```python
from build123d import *

# Parameters (mm, degrees)
SALIENTE_EXTRUIR1_DEPTH = 36.83
CROQUIS2_R              = 1.84
CROQUIS2_W              = 9.91
CROQUIS2_H              = 9.91
CORTAR_EXTRUIR1_DEPTH   = 49.541066699
CROQUIS3_W              = 2.1
CROQUIS3_H              = 17.6
CORTAR_EXTRUIR2_DEPTH   = 50.084125743


with BuildPart() as part:
    # Croquis1 → Saliente-Extruir1 (new body)
    with BuildSketch(Plane(origin=(0, 0, 0), x_dir=(0, 0, -1), z_dir=(1, 0, 0))):
        with BuildLine():
            Line((0, 0), (0, 19))
            ThreePointArc((0, 19), (-0.292893219, 19.707106781), (-1, 20))
            Line((-1, 20), (-5.045, 20))
            ThreePointArc((-5.045, 20), (-5.752106781, 19.707106781), (-6.045, 19))
            Line((-6.045, 19), (-6.045, 2.3725))
            ThreePointArc((-6.045, 2.3725), (-6.337893219, 1.665393219), (-7.045, 1.3725))
            Line((-7.045, 1.3725), (-18.505, 1.3725))
            ThreePointArc((-18.505, 1.3725), (-19.212106781, 1.665393219), (-19.505, 2.3725))
            Line((-19.505, 2.3725), (-19.505, 19))
            ThreePointArc((-19.505, 19), (-19.797893219, 19.707106781), (-20.505, 20))
            Line((-20.505, 20), (-24.55, 20))
            ThreePointArc((-24.55, 20), (-25.257106781, 19.707106781), (-25.55, 19))
            Line((-25.55, 19), (-25.55, 0))
            Line((-25.55, 0), (-24.1775, 0))
            Line((-24.1775, 0), (-24.1775, 17.6275))
            ThreePointArc((-24.1775, 17.6275), (-23.884606781, 18.334606781), (-23.1775, 18.6275))
            Line((-23.1775, 18.6275), (-21.8775, 18.6275))
            ThreePointArc((-21.8775, 18.6275), (-21.170393219, 18.334606781), (-20.8775, 17.6275))
            Line((-20.8775, 17.6275), (-20.8775, 1))
            ThreePointArc((-20.8775, 1), (-20.584606781, 0.292893219), (-19.8775, 0))
            Line((-19.8775, 0), (-5.6725, 0))
            ThreePointArc((-5.6725, 0), (-4.965393219, 0.292893219), (-4.6725, 1))
            Line((-4.6725, 1), (-4.6725, 17.6275))
            ThreePointArc((-4.6725, 17.6275), (-4.379606781, 18.334606781), (-3.6725, 18.6275))
            Line((-3.6725, 18.6275), (-2.3725, 18.6275))
            ThreePointArc((-2.3725, 18.6275), (-1.665393219, 18.334606781), (-1.3725, 17.6275))
            Line((-1.3725, 17.6275), (-1.3725, 0))
            Line((-1.3725, 0), (0, 0))
        make_face()
    extrude(amount=SALIENTE_EXTRUIR1_DEPTH)

    # Croquis2 → Cortar-Extruir1 (cut, through all)
    with BuildSketch(Plane(origin=(0, 1.3725, 0), x_dir=(1, 0, 0), z_dir=(0, 1, 0))):
        with Locations(Location((23.12, -12.775, 0), (0, 0, 270))):
            Circle(CROQUIS2_R)
        with Locations((4.955, -12.775)):
            Rectangle(CROQUIS2_W, CROQUIS2_H)
    extrude(amount=-CORTAR_EXTRUIR1_DEPTH, mode=Mode.SUBTRACT)

    # Croquis3 → Cortar-Extruir2 (cut, through all)
    with BuildSketch(Plane.XY.offset(25.55)):
        with Locations((5.44, 11.2)):
            Rectangle(CROQUIS3_W, CROQUIS3_H)
        with Locations((11.93, 11.2)):
            Rectangle(CROQUIS3_W, CROQUIS3_H)
        with Locations((18.42, 11.2)):
            Rectangle(CROQUIS3_W, CROQUIS3_H)
        with Locations((24.91, 11.2)):
            Rectangle(CROQUIS3_W, CROQUIS3_H)
        with Locations((31.4, 11.2)):
            Rectangle(CROQUIS3_W, CROQUIS3_H)
    extrude(amount=-CORTAR_EXTRUIR2_DEPTH, mode=Mode.SUBTRACT)


solid = part.part
```
CAD build for the part. Positions are in the model's coordinates, mm. A direction names the side the tool comes from. Coordinates: 2 decimals unless noted, no trailing zeros. Order: outer loops, then holes, each group sorted by start corner. A loop starts at its lowest first (then second) coordinate and runs counter-clockwise, first axis right, second up. Notation, with made-up numbers: M -26.5,-22 L -13.5,-22 A28 ccw -13.5,12 Z; hole C -8.5,-34 d7. An arc over 180 degrees is marked long. Answer as CSV lines item,"result".
1) 3-axis set-ups, long thin cutter, end or side, ignore diameter. For faces 1 (the flat face through (2, 20, 3)), 2 (the flat face through (31, 2.4, 20)), 3 (the cylindrical face through (21.634, 19.715, 25.249)), 4 (the cylindrical face through (21.634, 19.715, 5.744)), 5 (the cylindrical face through (15.144, 18.342, 21.178)): which of +Z, -Z, +X, -X, +Y, -Y reach the whole face in a straight line?
Verdict:
face 1,"+Z, -Z, +X, -X, +Y"
face 2,"+Z, -Z, +Y"
face 3,"+Z, +X, -X, +Y"
face 4,"+X, -X, +Y"
face 5,"+X, -X, -Y"
2) Mould opens along X. For faces 6 (the flat face through (36.83, 9, 20)), 7 (the flat face through (2, 18.628, 23)), 8 (the flat face through (32.45, 11, 25)) say: released by +X, released by -X, zero draft, split by the parting line, or undercut.
Verdict:
face 6,"released by +X"
face 7,"zero draft"
face 8,"undercut"
3) Cut at B-B (z = 3). List the corners of the cut face in (x, y).
Verdict:
outline,"M 0,18.63 L 4.39,18.63 L 4.39,20 L 0,20 Z; M 6.49,18.63 L 10.88,18.63 L 10.88,20 L 6.49,20 Z; M 12.98,18.63 L 17.37,18.63 L 17.37,20 L 12.98,20 Z; M 19.47,18.63 L 23.86,18.63 L 23.86,20 L 19.47,20 Z; M 25.96,18.63 L 30.35,18.63 L 30.35,20 L 25.96,20 Z; M 32.45,18.63 L 36.83,18.63 L 36.83,20 L 32.45,20 Z"
4) Cut at D-D (y = 8.5). Give the number of separate pieces and of enclosed holes in the cut face, then the cut area to 3 significant figures.
Verdict:
separate pieces,"24"
enclosed holes,"0"
area,"145 mm2"
5) Flat gauge pins, fed straight in: P1, Ø1.8, axis at y = 10, z = 1.5, coming from the +X side; P2, Ø12, axis at x = 13.5, z = 11.5, coming from the +Y side; P3, Ø4, axis at y = 12.5, z = 8.5, coming from the -X side. Where does each tip first touch, or does it go through?
Verdict:
P1,"x = 36.83"
P2,"y = 19.89"
P3,"through"
6) Drill centre lines: L1, parallel to Z at x = 35, y = 17.75 (3 decimals); L2, parallel to X at y = 8, z = 20.75; L3, parallel to Y at x = 24.5, z = 18. Where is each one in solid material? Low to high. Write a range as from..to.
Verdict:
L1,"0..1.38, 4.665..6.045, 19.505..20.885, 24.17..25.55"
L2,"0..4.39, 6.49..10.88, 12.98..17.37, 19.47..23.86, 25.96..30.35, 32.45..36.83"
L3,"0..1.37"
